Autodesk Fusion 360 part; units mm, degrees
sketch "Esquisse1" plane through (0, 0, 0) normal (0, 0, 1) x (1, 0, 0)
  line L0 (-22.5, 21.25) -> (22.5, 21.25)
  line L1 (22.5, 21.25) -> (22.5, -21.25)
  line L2 (22.5, -21.25) -> (-22.5, -21.25)
  line L3 (-22.5, -21.25) -> (-22.5, 21.25)
  line L4 (-22.5, 21.25) -> (22.5, -21.25) construction
  line L5 (22.5, 21.25) -> (-22.5, -21.25) construction
  line L6 (-22.5, 11.75) -> (-22.5, 21.25)
  line L7 (-22.5, -21.25) -> (-27.5, -21.25)
  line L8 (-27.5, -21.25) -> (-27.5, -16.25)
  line L9 (-27.5, -16.25) -> (-22.5, -16.25)
  line L10 (-22.5, -16.25) -> (-22.5, -21.25)
  line L11 (22.5, 21.25) -> (27.5, 21.25)
  line L12 (27.5, 21.25) -> (27.5, 16.25)
  line L13 (27.5, 16.25) -> (22.5, 16.25)
  line L14 (22.5, 16.25) -> (22.5, 21.25)
  line L15 (22.5, -21.25) -> (27.5, -21.25)
  line L16 (27.5, -21.25) -> (27.5, -16.25)
  line L17 (27.5, -16.25) -> (22.5, -16.25)
  line L18 (22.5, -16.25) -> (22.5, -21.25)
  line L19 (-20, -21.25) -> (20, -21.25)
  line L20 (20, -21.25) -> (20, 18.75)
  line L21 (20, 18.75) -> (-20, 18.75)
  line L22 (-20, 18.75) -> (-20, -21.25)
  line L23 (22.5, 21.25) -> (27.5, 16.25)
  line L24 (22.5, -16.25) -> (27.5, -21.25)
  line L25 (-27.5, -16.25) -> (-22.5, -21.25)
  circle A0 centre (25, 18.75) radius 1.9
  circle A1 centre (25, 18.75) radius 1
  circle A2 centre (25, -18.75) radius 1.9
  circle A3 centre (25, -18.75) radius 1
  circle A4 centre (-25, -18.75) radius 1.9
  circle A5 centre (-25, -18.75) radius 1
  line L26 (27.5, 21.25) -> (27.5, 16.25)
  circle A6 centre (25, 18.75) radius 1
  line L27 (-22.5, 21.25) -> (-27.5, 21.25)
  line L28 (-27.5, 21.25) -> (-27.5, 16.25)
  line L29 (-27.5, 16.25) -> (-22.5, 16.25)
  line L30 (-22.5, 16.25) -> (-22.5, 21.25)
  circle A7 centre (-25, 18.75) radius 1.9
  circle A8 centre (-25, 18.75) radius 1
  line L31 (-22.5, 16.25) -> (-27.5, 21.25)
  line L32 (27.5, 1.75) -> (22.5, 1.75)
  line L33 (22.5, 1.75) -> (27.5, -3.25)
  circle A9 centre (25, -0.75) radius 1
  circle A10 centre (25, -0.75) radius 1.9
  line L34 (27.5, -3.25) -> (27.5, 1.75)
  line L35 (22.5, -3.25) -> (27.5, -3.25)
  point P0 (25, 18.75)
  point P1 (-25, 18.75)
  dimension "d1" = 45
  dimension "d2" = 42.5
  dimension "d5" = 5
  dimension "d6" = 5
  dimension "d7" = 5
  dimension "d8" = 5
  dimension "d9" = 5
  dimension "d10" = 5
  dimension "d12" = 2.5
  dimension "d13" = 2.5
  dimension "d14" = 2.5
  dimension "d22" = 3.8
  dimension "d23" = 2
  dimension "d26" = 3.8
  dimension "d27" = 2
  dimension "d28" = 3.8
  dimension "d29" = 2
  dimension "d46" = 5
  dimension "d47" = 2
  dimension "d48" = 5
  dimension "d49" = 5
  dimension "d50" = 2
  dimension "d51" = 3.8
  dimension "d52" = 5
  dimension "d53" = 5
  dimension "d54" = 3.8
  dimension "d55" = 2
  dimension "d56" = 13
extrude "Extrusion1" add sketch "Esquisse1" along normal blind 24 contours L0 L1 L2 L3 L6 L10 L14 L18 L20 L21 L22 L30
extrude "Extrusion2" add sketch "Esquisse1" along normal blind 3 from surface at 21 contours L2 L19 L20 L21 L22
extrude "Extrusion3" add sketch "Esquisse1" along normal blind 5 contours L3 L6 L27 L30 A7 L31 | L28 L29 A7 L31 | A7 A8 L31 | A7 A8 L31 | L1 L33 A10 L35 | L32 L33 A10 L34 | L3 L9 L10 L25 A4 | A8 L31 | A8 L31 | L33 A9 A10 | L33 A9 A10 | L7 L8 L25 A4 | L33 A9 | L33 A9 | L25 A4 A5 | L25 A4 A5 | L25 A5 | L25 A5
extrude "Extrusion4" cut sketch "Esquisse1" against normal blind 2.5 from surface at 5 contours L23 A0 A1 A6 | L23 A0 A1 A6 | A7 A8 L31 | A7 A8 L31 | L33 A9 A10 | L33 A9 A10 | L25 A4 A5 | L25 A4 A5 | L24 A2 A3 | L24 A2 A3
extrude "Extrusion5" cut sketch "Esquisse1" along normal blind 8 contours A8 L31 | A8 L31 | L33 A9 | L33 A9 | L25 A5 | L25 A5 | L24 A3 | L24 A3
sketch "Esquisse2" plane through (-22.5, 0, 0) normal (-1, 0, 0) x (0, -1, 0)
  line L0 (16.25, 5) -> (21.25, 5)
  line L1 (21.25, 5) -> (21.25, 24)
  line L2 (21.25, 24) -> (-21.25, 24)
  line L3 (-21.25, 24) -> (-21.25, 5)
  line L4 (-16.25, 0) -> (16.25, 0)
  line L5 (16.25, 0) -> (16.25, 5)
  line L6 (-17.75, 0) -> (-17.75, 21)
  line L7 (-11.75, 0) -> (-11.75, 21)
  line L8 (-17.75, 21) -> (-11.75, 21)
  line L9 (-21.25, 5) -> (-16.25, 5)
  line L10 (-16.25, 5) -> (-16.25, 0)
  line L11 (-11.75, 0) -> (-17.75, 0)
  dimension "d35" = 3.5
  dimension "d36" = 6
  dimension "d37" = 21
  dimension "d38" = 21
extrude "Extrusion6" cut sketch "Esquisse2" against normal blind 9 from surface at -40 contours L4 L6 L7 L8 L9 L10 L11 | L6 L9 L10 L11
sketch "Esquisse3" plane through (22.5, 0, 0) normal (1, 0, 0) x (0, 1, 0)
  line L0 (17.75, 0) -> (21.25, 0)
  line L1 (21.25, 0) -> (21.25, 24)
  line L2 (17.75, 0) -> (27.75, 0)
  line L3 (27.75, 0) -> (27.75, 21)
  line L4 (27.75, 21) -> (17.75, 21)
  line L5 (17.75, 21) -> (17.75, 0)
  line L6 (17.75, 21) -> (17.75, 0)
  line L7 (11.75, 0) -> (11.75, 21)
  line L8 (11.75, 21) -> (17.75, 21)
  line L9 (21.25, 24) -> (-21.25, 24)
  line L10 (-21.25, 24) -> (-21.25, 0)
  line L11 (-3.25, 5) -> (1.75, 5)
  line L12 (1.75, 0) -> (11.75, 0)
  line L13 (-21.25, 0) -> (-3.25, 0)
  line L14 (-3.25, 0) -> (-3.25, 5)
  line L15 (1.75, 5) -> (1.75, 0)
  dimension "d41" = 10
  dimension "d42" = 21
Check sheet for the modelled part. Datum: model origin and axes. Units: mm. A direction names the side the tool comes from. Give positions to 0.01 mm unless a question says otherwise; leave off trailing zeros. Order: outer loops, then holes, each group sorted by start corner. A loop starts at its lowest first (then second) coordinate and runs counter-clockwise, first axis right, second up. Notation, with made-up numbers: (7.5, -23.5) -> (17.5, -23.5) arc R18 cw to (17.5, -5.5) -> close; hole circle Ø10 at (-25.75, 44). An arc over 180 degrees is marked (long way). Return JSON: item names as keys, results as strings.
1. Cross-section at B-B, the plane x = -25. Record the cut outline in (y, z).
From the geometry:
{"outline": "(-21.25, 0) -> (-19.75, 0) -> (-19.75, 2.5) -> (-20.65, 2.5) -> (-20.65, 5) -> (-21.25, 5) -> close; (-17.75, 0) -> (-16.25, 0) -> (-16.25, 5) -> (-16.85, 5) -> (-16.85, 2.5) -> (-17.75, 2.5) -> close; (16.25, 0) -> (17.75, 0) -> (17.75, 2.5) -> (16.85, 2.5) -> (16.85, 5) -> (16.25, 5) -> close; (19.75, 0) -> (21.25, 0) -> (21.25, 5) -> (20.65, 5) -> (20.65, 2.5) -> (19.75, 2.5) -> close"}
2. Cross-section at A-A, the plane z = 4. Record the cut outline in (x, y), plus the area to 3 significant figures.
From the geometry:
{"outline": "(-27.5, -21.25) -> (-20, -21.25) -> (-20, 18.75) -> (20, 18.75) -> (20, 17.75) -> (22.5, 17.75) -> (22.5, 21.25) -> (-27.5, 21.25) -> (-27.5, 16.25) -> (-22.5, 16.25) -> (-22.5, -16.25) -> (-27.5, -16.25) -> close; (20, -21.25) -> (22.5, -21.25) -> (22.5, -3.25) -> (27.5, -3.25) -> (27.5, 1.75) -> (22.5, 1.75) -> (22.5, 11.75) -> (20, 11.75) -> close; hole circle Ø3.8 at (-25, -18.75); hole circle Ø3.8 at (-25, 18.75); hole circle Ø3.8 at (25, -0.75)", "area": "338 mm^2"}
3. Mould release check, pull along Y, two halves, no side actions. Record for faces 5 (the cylindrical face through (-26.4, 20.034, 3.768)), 6 (the flat face through (-20, -1, 10)): +Y half, -Y half, draft (parallel to the pull), parting line (faces both ways), or undercut.
From the geometry:
{"face 5": "undercut", "face 6": "draft"}
4. Cross-section at D-D, the plane x = 25. Record the cut outline in (y, z).
From the geometry:
{"outline": "(-3.25, 0) -> (-1.75, 0) -> (-1.75, 2.5) -> (-2.65, 2.5) -> (-2.65, 5) -> (-3.25, 5) -> close; (0.25, 0) -> (1.75, 0) -> (1.75, 5) -> (1.15, 5) -> (1.15, 2.5) -> (0.25, 2.5) -> close"}
5. Cross-section at C-C, the plane z = 10.25. Record the cut outline in (x, y).
From the geometry:
{"outline": "(-22.5, -21.25) -> (-20, -21.25) -> (-20, 18.75) -> (20, 18.75) -> (20, 17.75) -> (22.5, 17.75) -> (22.5, 21.25) -> (-22.5, 21.25) -> close; (20, -21.25) -> (22.5, -21.25) -> (22.5, 11.75) -> (20, 11.75) -> close"}
6. Material ranges on probe 1 along X at (y, z) = (-0.75, 3.6); probe 2 along X at (y, z) = (-18.75, 3.9); probe 3 along Y at (x, z) = (-25, 4.35), recorded low to high. Write a range as [from, to].
From the geometry:
{"probe 1": "[-22.5, -20], [20, 23.1], [26.9, 27.5]", "probe 2": "[-27.5, -26.9], [-23.1, -20], [20, 22.5]", "probe 3": "[-21.25, -20.65], [-16.85, -16.25], [16.25, 16.85], [20.65, 21.25]"}
7. Set-up check for faces 1 (the cylindrical face through (23.492, -1.906, 3.768)), 2 (the flat face through (27, -2, 5)), 3 (the flat face through (21, 11.75, 10)), 4 (the flat face through (-25, -16.25, 2)): record each of +Z, -Z, +X, -X, +Y, -Y from which the full face is reachable in a straight line by a thin tool's end or side.
From the geometry:
{"face 1": "+Z", "face 2": "+Z, +X, +Y, -Y", "face 3": "-Z, +X", "face 4": "+Z, -Z, -X"}
8. Go/stop test with flat-tipped pins: P1, Ø3.5, axis at x = -25, y = 18.75, coming from the +Z side; P2, Ø3, axis at x = 25.5, y = 0, coming from the +Z side; P3, Ø1.5, axis at y = -3.5, z = 10.5, coming from the +X side. Record where each tip stops, or that it passes through.
From the geometry:
{"P1": "z = 2.5", "P2": "z = 5", "P3": "x = 22.5"}
